The listing builds one solid part. Answer for the finished solid, in the listing's coordinates (mm). Face numbers are marked on the shaded views. A direction names the side the tool comes from. Coordinates: 2 decimals unless noted, no trailing zeros. Loops run counter-clockwise (first coordinate to the right, second up) from the corner with the lowest first, then second, coordinate; pieces in that order, holes last. Notation, with made-up numbers: M 70.25,79 L 75.25,79 A5 ccw 75.25,85 Z; hole C 8,40 d9. An arc over 180 degrees is marked long. Return JSON: item names as keys, results as strings. Group by question number.
1. Section B-B (x = 33) is taken. Write down the section's boundary in (y, z), then the cut area to 3 significant figures.
2. Given P1, Ø2, axis at x = -14, y = 13, coming from the -Z side, flat-ended and moving along its own axis, determine where the tip first touches the part or whether it passes through.
3. Section D-D (z = -4.5) is taken. Write down the section's boundary in (x, y) (3 decimals).
4. The mould has two halves that part along Y. Classify the marked faces 3, 4, 5 and 6: pulls with the +Y half, pulls with the -Y half, needs draft (parallel to the pull), parting line crosses it, or undercut.
5. Section C-C (y = 11.5) is taken. Write down the section's boundary in (x, z), then the cut area to 3 significant figures.
6. Which of the six approach directions +Z, -Z, +X, -X, +Y, -Y give full straight-line access (tool end or side, diameter ignored) to the marked faces 1 and 2?
7. Section A-A (y = 0) is taken. Write down the section's boundary in (x, z), then the cut area to 3 significant figures.
8. Straight lines are drawn through the part: L1, parallel to X at y = -9, z = 0.75; L2, parallel to Y at x = -25.5, z = 6; L3, parallel to X at y = 11, z = -4. For each, find the intervals that lie inside material, in ascending order. Write a range as from..to.
```python
from build123d import *

# Parameters (mm, degrees)
SKETCH1_W               = 83.4898
SKETCH1_H               = 38.1
BOSS_EXTRUDE1_DEPTH     = 6.35
SKETCH2_W               = 25.4
SKETCH2_H               = 38.1
BOSS_EXTRUDE2_DEPTH     = 7.4549
CUT_EXTRUDE1_DEPTH      = 48.917788347
CUT_EXTRUDE1_DEPTH_BACK = 48.917788347
SKETCH6_R               = 4.826
SKETCH8_R               = 4.826
CUT_EXTRUDE2_DEPTH      = 48.917788347
FILLET1_R               = 2.54


with BuildPart() as part:
    # Sketch1 → Boss-Extrude1 (new body)
    with BuildSketch(Plane.XY):
        Rectangle(SKETCH1_W, SKETCH1_H)
    extrude(amount=BOSS_EXTRUDE1_DEPTH)

    # Sketch2 → Boss-Extrude2 (add)
    with BuildSketch(Plane(origin=(0, 0, 0), x_dir=(-1, 0, 0), z_dir=(0, 0, -1))):
        with Locations((-29.0449, 0)):
            Rectangle(SKETCH2_W, SKETCH2_H)
    extrude(amount=BOSS_EXTRUDE2_DEPTH)

    # Sketch6 → Cut-Extrude1 (cut, two sides: drawn at the far end of the back side and taken through both)
    with BuildSketch(Plane(origin=(0, 0, -7.4549), x_dir=(-1, 0, 0), z_dir=(0, 0, -1)).offset(-CUT_EXTRUDE1_DEPTH_BACK)):
        with Locations((-29.0449, 9.525)):
            Circle(SKETCH6_R)
        with Locations((-29.0449, -9.525)):
            Circle(SKETCH6_R)
    extrude(amount=CUT_EXTRUDE1_DEPTH + CUT_EXTRUDE1_DEPTH_BACK, mode=Mode.SUBTRACT)

    # Sketch8 → Cut-Extrude2 (cut, through all)
    with BuildSketch(Plane.XY.offset(6.35)):
        with Locations((-29.0449, -9.525)):
            Circle(SKETCH8_R)
        with Locations((-29.0449, 9.525)):
            Circle(SKETCH8_R)
    extrude(amount=-CUT_EXTRUDE2_DEPTH, mode=Mode.SUBTRACT)

    # Fillet1
    fillet1_edges = [part.edges().sort_by_distance(p)[0] for p in [
        (-41.7449, 0, 6.35),
        (41.7449, 0, 6.35),
    ]]
    fillet(fillet1_edges, radius=FILLET1_R)


solid = part.part
```
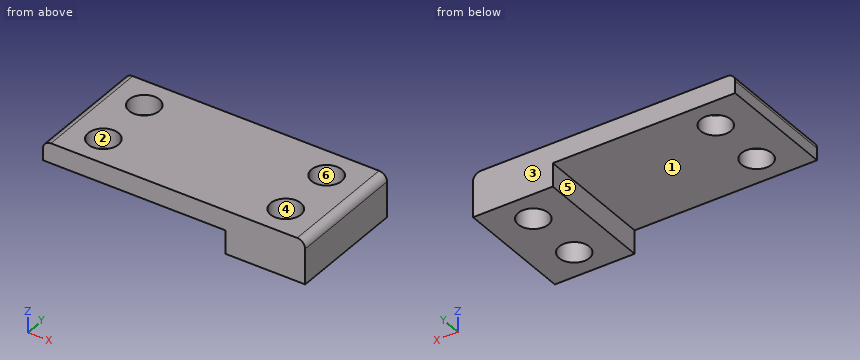
Worked out:
{
 "1": {"outline": "M -19.05,-7.45 L -12.29,-7.45 L -12.29,6.35 L -19.05,6.35 Z; M -6.76,-7.45 L 6.76,-7.45 L 6.76,6.35 L -6.76,6.35 Z; M 12.29,-7.45 L 19.05,-7.45 L 19.05,6.35 L 12.29,6.35 Z", "area": "373 mm^2"},
 "2": {"P1": "z = 0"},
 "3": {"outline": "M 16.345,-19.05 L 41.745,-19.05 L 41.745,19.05 L 16.345,19.05 Z; hole C 29.045,-9.525 d9.652; hole C 29.045,9.525 d9.652"},
 "4": {"face 3": "pulls with the +Y half", "face 4": "undercut", "face 5": "needs draft", "face 6": "undercut"},
 "5": {"outline": "M -41.74,0 L -33.45,0 L -33.45,6.35 L -39.2,6.35 A2.54 ccw -41.74,3.81 Z; M -24.64,0 L 16.34,0 L 16.34,-7.45 L 24.64,-7.45 L 24.64,6.35 L -24.64,6.35 Z; M 33.45,-7.45 L 41.74,-7.45 L 41.74,3.81 A2.54 ccw 39.2,6.35 L 33.45,6.35 Z", "area": "539 mm^2"},
 "6": {"face 1": "-Z, -X, +Y, -Y", "face 2": "+Z, -Z"},
 "7": {"outline": "M -41.74,0 L 16.34,0 L 16.34,-7.45 L 41.74,-7.45 L 41.74,3.81 A2.54 ccw 39.2,6.35 L -39.2,6.35 A2.54 ccw -41.74,3.81 Z", "area": "717 mm^2"},
 "8": {"L1": "-41.74..-33.84, -24.25..24.25, 33.84..41.74", "L2": "-19.05..-12.8, -6.25..6.25, 12.8..19.05", "L3": "16.34..24.45, 33.64..41.74"}
}
